```python
from build123d import *

# Parameters (mm, degrees)
ESQUISSE1_W        = 5
ESQUISSE1_H        = 5
BOSS_EXTRU_1_DEPTH = 5
D_GAGEMENT_M41_D   = 4.5


with BuildPart() as part:
    # Esquisse1 → Boss.-Extru.1 (new body)
    with BuildSketch(Plane.XY):
        with BuildLine():
            Line((-58.909278233, -55), (-63.909278233, -55))
            ThreePointArc((-63.909278233, -55), (-70.980346045, -52.071067812), (-73.909278233, -45))
            Line((-73.909278233, -45), (-73.909278233, 45))
            ThreePointArc((-73.909278233, 45), (-70.980346045, 52.071067812), (-63.909278233, 55))
            Line((-63.909278233, 55), (-58.909278233, 55))
            ThreePointArc((-58.909278233, 55), (-55.373744327, 53.535533906), (-53.909278233, 50))
            Line((-53.909278233, 50), (-53.909278233, 32.9))
            ThreePointArc((-53.909278233, 32.9), (-52.444812139, 29.364466094), (-48.909278233, 27.9))
            Line((-48.909278233, 27.9), (-25.4, 27.9))
            ThreePointArc((-25.4, 27.9), (-7.439487758, 20.460512242), (0, 2.5))
            Line((0, 2.5), (-10, 2.5))
            ThreePointArc((-10, 2.5), (-13.202056301, 3.42586604), (-15.41588754, 5.917721519))
            ThreePointArc((-15.41588754, 5.917721519), (-41.577296486, 0), (-15.41588754, -5.917721519))
            ThreePointArc((-15.41588754, -5.917721519), (-13.202056301, -3.42586604), (-10, -2.5))
            Line((-10, -2.5), (0, -2.5))
            ThreePointArc((0, -2.5), (-7.439487758, -20.460512242), (-25.4, -27.9))
            Line((-25.4, -27.9), (-48.909278233, -27.9))
            ThreePointArc((-48.909278233, -27.9), (-52.444812139, -29.364466094), (-53.909278233, -32.9))
            Line((-53.909278233, -32.9), (-53.909278233, -50))
            ThreePointArc((-53.909278233, -50), (-55.373744327, -53.535533906), (-58.909278233, -55))
        make_face()
        with Locations((-27.827296486, 20.4)):
            Rectangle(ESQUISSE1_W, ESQUISSE1_H, mode=Mode.SUBTRACT)
        Polygon((-9.245314739, 13.615063509), (-6.745314739, 9.284936491), (-11.075441758, 6.784936491), (-13.575441758, 11.115063509), align=None, mode=Mode.SUBTRACT)
        Polygon((-6.745314739, -9.284936491), (-9.245314739, -13.615063509), (-13.575441758, -11.115063509), (-11.075441758, -6.784936491), align=None, mode=Mode.SUBTRACT)
        with Locations((-27.827296486, -20.4)):
            Rectangle(ESQUISSE1_W, ESQUISSE1_H, mode=Mode.SUBTRACT)
        Polygon((-46.409278233, -13.615063509), (-48.909278233, -9.284936491), (-44.579151214, -6.784936491), (-42.079151214, -11.115063509), align=None, mode=Mode.SUBTRACT)
        Polygon((-48.909278233, 9.284936491), (-46.409278233, 13.615063509), (-42.079151214, 11.115063509), (-44.579151214, 6.784936491), align=None, mode=Mode.SUBTRACT)
    extrude(amount=BOSS_EXTRU_1_DEPTH)

    # Dégagement M41 (through all)
    with Locations(Plane.XY.offset(5)):
        with Locations((-63.909278233, 45), (-63.909278233, -45)):
            Hole(D_GAGEMENT_M41_D / 2)


solid = part.part
```
CAD build for the part. Positions are in the model's coordinates, mm. A direction names the side the tool comes from. Round coordinates to 2 decimals unless told otherwise and drop trailing zeros. Order: outer loops, then holes, each group sorted by start corner. A loop starts at its lowest first (then second) coordinate and runs counter-clockwise, first axis right, second up. Notation, with made-up numbers: (76.25, -25.5) - (86.25, -25.5) arc R11 ccw to (86.25, -4.5) - close; hole circle Ø3 at (73.5, 62). An arc over 180 degrees is marked (long way). Use CSV: the item, a comma, the result in double quotes. Start each with the question number.
1) Pin check, flat tips, straight feed: pin 1 Ø2.5 at (x, z) = (-27.5, 3) entering from +Y; pin 2 Ø16.5 at (x, y) = (-27.83, 0) entering from +Z; pin 3 Ø1.5 at (y, z) = (-41.5, 2.5) entering from +X; pin 4 Ø2.5 at (x, z) = (-32, 3) entering from -Y. Stop position of each tip, or through.
2) Two-plate mould, pull along X, no slides. Class faces 1 (the flat face through (-37, -27.9, 2)), 2 (the flat face through (-47.677, 11.42, 2.465)), 3 (the flat face through (-7.98, -11.42, 2.46)), 4 (the cylindrical face through (-7.24, -20.26, 2.46)): pulls with the +X half, pulls with the -X half, needs draft (parallel to the pull), parting line crosses it, or undercut.
3) Saw through at A-A (x = -22). List the corners of the cut face in (y, z), and give its area (3 significant figures).
4) Saw through at C-C (y = 0). List the corners of the cut face in (x, z).
5) Saw through at B-B (y = -20.5). List the corners of the cut face in (x, z).
6) Wall check: L1, parallel to Y at x = -64.5, z = 4.1; L2, parallel to Y at x = -44.5, z = 2.1; L3, parallel to X at y = 8, z = 0.65. Give the ranges that are in metal, low to high. Write a range as [from, to].
7) Saw through at D-D (z = 2.5). Count the separate pieces of the cut face and the enclosed holes in it, and give its area (3 significant figures).
8) Tool access for faces 5 (the flat face through (-30.327, -20, 2)), 6 (the cylindrical face through (-52.41, -29.33, 2.46)): list every direction of +Z, -Z, +X, -X, +Y, -Y with a clear straight run to the whole face (end or side of a thin tool).
Values follow:
1,pin 1,"stops at y = 27.9"
1,pin 2,"passes through"
1,pin 3,"stops at x = -53.91"
1,pin 4,"stops at y = -27.9"
2,face 1,"needs draft"
2,face 2,"undercut"
2,face 3,"undercut"
2,face 4,"pulls with the +X half"
3,outline,"(-27.67, 0) - (-12.45, 0) - (-12.45, 5) - (-27.67, 5) - close; (12.45, 0) - (27.67, 0) - (27.67, 5) - (12.45, 5) - close"
3,area,"152 mm2"
4,outline,"(-73.91, 0) - (-41.58, 0) - (-41.58, 5) - (-73.91, 5) - close"
5,outline,"(-73.91, 0) - (-30.33, 0) - (-30.33, 5) - (-73.91, 5) - close; (-25.33, 0) - (-7.48, 0) - (-7.48, 5) - (-25.33, 5) - close"
6,L1,"y = [-54.98, -47.17], [-42.83, 42.83], [47.17, 54.98]"
6,L2,"y = [-27.9, -12.51], [-6.92, 6.92], [12.51, 27.9]"
6,L3,"x = [-73.91, -46.68], [-43.88, -39.01], [-16.64, -11.78], [-8.97, -0.6]"
7,separate pieces,"1"
7,enclosed holes,"8"
7,area,"4,040 mm2"
8,face 5,"+Z, -Z"
8,face 6,"+Z, -Z, +X, -Y"
